from build123d import *

# Parameters (mm, degrees)
F0_W          = 54
F0_H          = 45
F0_W_2        = 44
F0_H_2        = 35
F1_DEPTH      = 40
F2_DEPTH      = 5
F3_W          = 6
F3_H          = 45
F4_DEPTH      = 70
F6_R          = 5
F7_DEPTH      = 40
F5_R          = 4
F8_DEPTH      = 48.001
F8_DEPTH_BACK = 25
F9_DEPTH      = 20
F10_DEPTH     = 6


with BuildPart() as f1:
    # F0 (on Top) → F1 (new body)
    with BuildSketch(Plane.XY):
        Rectangle(F0_W, F0_H)
        Rectangle(F0_W_2, F0_H_2, mode=Mode.SUBTRACT)
    extrude(amount=-F1_DEPTH)

    # F0 (on Top) → F2 (join)
    with BuildSketch(Plane.XY):
        Rectangle(F0_W, F0_H)
        Rectangle(F0_W_2, F0_H_2, mode=Mode.SUBTRACT)
        Rectangle(F0_W_2, F0_H_2)
    extrude(amount=F2_DEPTH)

    # F3 (on face) → F4 (join)
    with BuildSketch(Plane.XY.offset(5)):
        with Locations((24, 0)):
            Rectangle(F3_W, F3_H)
        with Locations((-24, 0)):
            Rectangle(F3_W, F3_H)
    extrude(amount=F4_DEPTH)

    # F6
    f6_edges = [f1.edges().sort_by_distance(p)[0] for p in [
        (-24, -22.5, 75),
        (-24, 22.5, 75),
        (24, -22.5, 75),
        (24, 22.5, 75),
        (27, -22.5, 17.5),
        (27, 0, 75),
        (27, 22.5, 17.5),
        (-27, -22.5, 17.5),
        (-27, 22.5, 17.5),
        (-27, 0, 75),
    ]]
    fillet(f6_edges, radius=F6_R)

    # F7 (add): a face of the model
    f7_faces = [f1.faces().sort_by_distance(p)[0] for p in [
        (0, 0, 5),
    ]]
    extrude(f7_faces, amount=F7_DEPTH)

    # F5 (on face) → F8 (cut, two sides)
    with BuildSketch(Plane.YZ.offset(-21)) as f8_sk:
        with Locations((-13.5, 65)):
            Circle(F5_R)
    extrude(amount=F8_DEPTH, mode=Mode.SUBTRACT)
    extrude(f8_sk.sketch, amount=-F8_DEPTH_BACK, mode=Mode.SUBTRACT)

    # F9 (add): a face of the model
    f9_faces = [f1.faces().sort_by_distance(p)[0] for p in [
        (-21, 0.526440406, 59.6894541328),
    ]]
    extrude(f9_faces, amount=F9_DEPTH)

    # F10 (add): a face of the model
    f10_faces = [f1.faces().sort_by_distance(p)[0] for p in [
        (21, 0.526440406, 59.6894541328),
    ]]
    extrude(f10_faces, amount=F10_DEPTH)


solid = f1.part
Design review of the part built by this model. Coordinates are the model's own, in mm. A direction names the side the tool comes from. Round coordinates to 2 decimals unless told otherwise and drop trailing zeros. Write each loop counter-clockwise with the first axis right and the second up, starting at its lowest first coordinate (ties: lowest second). Pieces come first, ordered by that corner, then holes.
Item 1: Draft analysis for pull direction Y (two halves, no side actions). For faces 4 (the cylindrical face through (-11.65, 21, 73.57)), 5 (the cylindrical face through (18.55, -21, 73.57)), 6 (the flat face through (22, 0, -20)), state which applies: released by +Y, released by -Y, zero draft, split by the parting line, or undercut.
Item 2: Wall thickness on L1, parallel to Z at x = -22.5, y = -13.5; L2, parallel to X at y = 13.5, z = -4; L3, parallel to Z at x = -7.5, y = -13.5: over which ranges is each line inside the solid? List them lowest first.
Item 3: For faces 1 (the flat face through (-1, 0, 60)), 2 (the flat face through (0, 22.5, 14)), 3 (the flat face through (0, 17.5, -20)), list the 3-axis set-ups (+Z, -Z, +X, -X, +Y, -Y) from which the entire face can be reached by the end or side of a thin tool; tool diameter is ignored.
Item 4: Consider section C-C on z = 67.5. Give the boundary of the cut face in (x, y), and give its area (3 significant figures).
Item 5: For pin 1 Ø7 at (y, z) = (-13.5, 65) entering from -X; pin 2 Ø13 at (x, y) = (7.5, 10) entering from +Z; pin 3 Ø10.5 at (x, y) = (7.5, 4.5) entering from -Z, all flat-tipped, find the tip position at first contact; note any pin that passes through.
Item 6: Consider section A-A on x = -4.5. Give the boundary of the cut face in (y, z), and give its area (3 significant figures).
Item 7: Consider section D-D on x = 11. Give the boundary of the cut face in (y, z).
Item 8: Consider section B-B on y = -13.5. Give the boundary of the cut face in (x, z).
Check values:
1. face 4: released by +Y
1. face 5: released by -Y
1. face 6: undercut
2. L1: z = -40 to 61, 69 to 74.97
2. L2: x = -27 to -22, 22 to 27
2. L3: z = 0 to 61, 69 to 75
3. face 1: +Z, +Y, -Y
3. face 2: +Z, -Z, +X, -X, +Y
3. face 3: -Z
4. outline: (-27, -17.5) arc R5 ccw to (-22, -22.5) - (-1, -22.5) - (-1, -16.62) - (-27, -16.62) - close; (-27, -10.38) - (-1, -10.38) - (-1, 22.5) - (-22, 22.5) arc R5 ccw to (-27, 17.5) - close; (15, -22.5) - (22, -22.5) arc R5 ccw to (27, -17.5) - (27, -16.62) - (15, -16.62) - close; (15, -10.38) - (27, -10.38) - (27, 17.5) arc R5 ccw to (22, 22.5) - (15, 22.5) - close
4. area: 1,450 mm2
5. pin 1: passes through
5. pin 2: stops at z = 45
5. pin 3: stops at z = 0
6. outline: (-22.5, -40) - (-17.5, -40) - (-17.5, 0) - (17.5, 0) - (17.5, -40) - (22.5, -40) - (22.5, 70) arc R5 ccw to (17.5, 75) - (-17.5, 75) arc R5 ccw to (-22.5, 70) - close; hole circle Ø8 at (-13.5, 65)
6. area: 3,710 mm2
7. outline: (-22.5, -40) - (-17.5, -40) - (-17.5, 0) - (17.5, 0) - (17.5, -40) - (22.5, -40) - (22.5, 45) - (-22.5, 45) - close
8. outline: (-27, -40) - (-22, -40) - (-22, 0) - (22, 0) - (22, -40) - (27, -40) - (27, 61) - (15, 61) - (15, 45) - (-1, 45) - (-1, 61) - (-27, 61) - close; (-27, 69) - (-1, 69) - (-1, 75) - (-22, 75) arc R5 ccw to (-27, 70) - close; (15, 69) - (27, 69) - (27, 70) arc R5 ccw to (22, 75) - (15, 75) - close
